```python
from build123d import *

# Parameters (mm, degrees)
SKETCH1_W           = 10
SKETCH1_H           = 10
BOSS_EXTRUDE1_DEPTH = 10
SKETCH2_R           = 3
CUT_EXTRUDE1_DEPTH  = 10
FILLET2_R           = 5
SKETCH3_W           = 20
SKETCH3_H           = 10
BOSS_EXTRUDE3_DEPTH = 15
CUT_EXTRUDE2_DEPTH  = 15
SKETCH5_W           = 10
SKETCH5_H           = 20
BOSS_EXTRUDE4_DEPTH = 3
CUT_EXTRUDE3_DEPTH  = 10


with BuildPart() as part:
    # Sketch1 → Boss-Extrude1 (new body)
    with BuildSketch(Plane.XY):
        with Locations((1.321243523, -0.103626943)):
            Rectangle(SKETCH1_W, SKETCH1_H)
    extrude(amount=BOSS_EXTRUDE1_DEPTH)

    # Sketch2 → Cut-Extrude1 (cut)
    with BuildSketch(Plane(origin=(6.321243523, 0, 0), x_dir=(0, 0, -1), z_dir=(1, 0, 0))):
        with Locations(Location((-5, -0.103626943, 0), (0, 0, 90))):
            Circle(SKETCH2_R)
    extrude(amount=-CUT_EXTRUDE1_DEPTH, mode=Mode.SUBTRACT)

    # Fillet2
    fillet2_edges = [part.edges().sort_by_distance(p)[0] for p in [
        (1.321243523, -5.103626943, 0),
        (1.321243523, 4.896373057, 0),
    ]]
    fillet(fillet2_edges, radius=FILLET2_R - 0.0001)  # a hair under: the kernel refuses the full size

    # Sketch3 → Boss-Extrude3 (add)
    with BuildSketch(Plane.XY.offset(10)):
        with Locations((1.321243523, -0.103626943)):
            Rectangle(SKETCH3_W, SKETCH3_H)
    extrude(amount=BOSS_EXTRUDE3_DEPTH)

    # Sketch4 → Cut-Extrude2 (cut)
    with BuildSketch(Plane(origin=(0, 4.896373057, 0), x_dir=(1, 0, 0), z_dir=(0, 1, 0))):
        Polygon((11.321243523, -17.5), (6.321243523, -25), (11.321243523, -25), align=None)
        Polygon((-8.678756477, -25), (-3.678756477, -25), (-8.678756477, -17.5), align=None)
    extrude(amount=-CUT_EXTRUDE2_DEPTH, mode=Mode.SUBTRACT)

    # Sketch5 → Boss-Extrude4 (add)
    with BuildSketch(Plane(origin=(0, 4.896373057, 0), x_dir=(1, 0, 0), z_dir=(0, 1, 0))):
        with Locations((1.321243523, -15)):
            Rectangle(SKETCH5_W, SKETCH5_H)
    extrude(amount=BOSS_EXTRUDE4_DEPTH)

    # Sketch6 → Cut-Extrude3 (cut)
    with BuildSketch(Plane.ZY.offset(3.678756477)):
        Polygon((17.5, 7.896373057), (25, 4.896373057), (25, 7.896373057), align=None)
    extrude(amount=-CUT_EXTRUDE3_DEPTH, mode=Mode.SUBTRACT)


solid = part.part
```
For this review, take the finished solid that the model builds, in its own axes (mm). A direction names the side the tool comes from. Give positions to 0.01 mm unless a question says otherwise; leave off trailing zeros. Order: outer loops, then holes, each group sorted by start corner. A loop starts at its lowest first (then second) coordinate and runs counter-clockwise, first axis right, second up.
1) Take a section at B-B (z = 12.75). Give the boundary of the cut face in (x, y), then the cut area to 3 significant figures.
2) For faces 1 (the face through (-6, 4.896, 16)), 2 (the face through (1, 6, 5)), 3 (the face through (9, 0, 10)), list the 3-axis set-ups (+Z, -Z, +X, -X, +Y, -Y) from which the entire face can be reached by the end or side of a thin tool; tool diameter is ignored.
3) Take a section at D-D (x = 7.5). Give the boundary of the cut face in (y, z), then the cut area to 3 significant figures.
4) Take a section at C-C (y = 1.5). Give the boundary of the cut face in (x, z).
5) Wall thickness on line 1 (Z direction, x = -2, y = -0.25); line 2 (Z direction, x = 4, y = 0.5); line 3 (Y direction, x = 9.5, z = 15.75): over which ranges is each line inside the solid? List them lowest first.
6) Insertion check: pin 1 (2 mm diameter, centred on x = 3, y = -3, fed in from -Z); pin 2 (6 mm diameter, centred on x = -0.5, y = 3, fed in from -Z); pin 3 (1.5 mm diameter, centred on x = -0.5, y = 6, fed in from -Z); pin 4 (4 mm diameter, centred on x = 9.5, z = 21, fed in from +Y). Each pin has a flat end and moves straight along its axis. Give the tip position at first contact, or say it passes through.
7) The part is to be moulded in two halves that separate along Y. For faces 4 (the face through (1, 0, 25)), 5 (the face through (1.39, -0.75, 2.07)), 6 (the face through (1.251, 6.417, 21.198)), 7 (the face through (1.391, -3.678, 1.504)), say which applies: released by +Y, released by -Y, zero draft, split by the parting line, or undercut.
Derived:
1. outline: (-8.68, -5.1) - (11.32, -5.1) - (11.32, 4.9) - (6.32, 4.9) - (6.32, 7.9) - (-3.68, 7.9) - (-3.68, 4.9) - (-8.68, 4.9) - close
1. area: 230 mm2
2. face 1: +Z, -Z, -X, +Y
2. face 2: -Z, +X, -X, +Y
2. face 3: -Z, +X, +Y, -Y
3. outline: (-5.1, 10) - (4.9, 10) - (4.9, 23.23) - (-5.1, 23.23) - close
3. area: 132 mm2
4. outline: (-8.68, 10) - (-3.68, 10) - (-3.68, 7.54) - (6.32, 7.54) - (6.32, 10) - (11.32, 10) - (11.32, 17.5) - (6.32, 25) - (-3.68, 25) - (-8.68, 17.5) - close; (-3.68, 0.26) - (6.32, 0.26) - (6.32, 2.46) - (-3.68, 2.46) - close
5. line 1: z = 0 to 2, 8 to 25
5. line 2: z = 0.04 to 2.06, 7.94 to 25
5. line 3: y = -5.1 to 4.9
6. pin 1: stops at z = 0.37
6. pin 2: stops at z = 0
6. pin 3: stops at z = 5
6. pin 4: stops at y = 4.9
7. face 4: zero draft
7. face 5: undercut
7. face 6: released by +Y
7. face 7: released by -Y
